For this review, use the dimensioned drawing (mm, ordinates from the lowest corner) and the shaded views. Coordinates: 2 decimals unless noted, no trailing zeros. Order: outer loops, then holes, each group sorted by start corner. A loop starts at its lowest first (then second) coordinate and runs counter-clockwise, first axis right, second up. Notation, with made-up numbers: (-33, -38.5) -> (10, -38.5) arc R31 cw to (10, -3.5) -> close; hole circle Ø9 at (64, -7). An arc over 180 degrees is marked (long way). Use one line per item in the form item = value. Start each with the question number.
(1) Take a section at A-A (z = 13.75). State the section outline as (x, y) points, then the cut area to 3 significant figures.
(2) Wall thickness on line 1 along X through (y, z) = (4, 24); line 2 along Z through (x, y) = (1.6, 4.6); line 3 along X through (y, z) = (1.9, 4.75): over which ranges is each line inside the solid? List them lowest first.
(3) Insertion check: pin 1 Ø3 at (y, z) = (2, 14.5) entering from -X; pin 2 Ø1 at (x, z) = (1.5, 21) entering from -Y. Each pin has a flat end and moves straight along its axis. Give the tip position at first contact, or say it passes through.
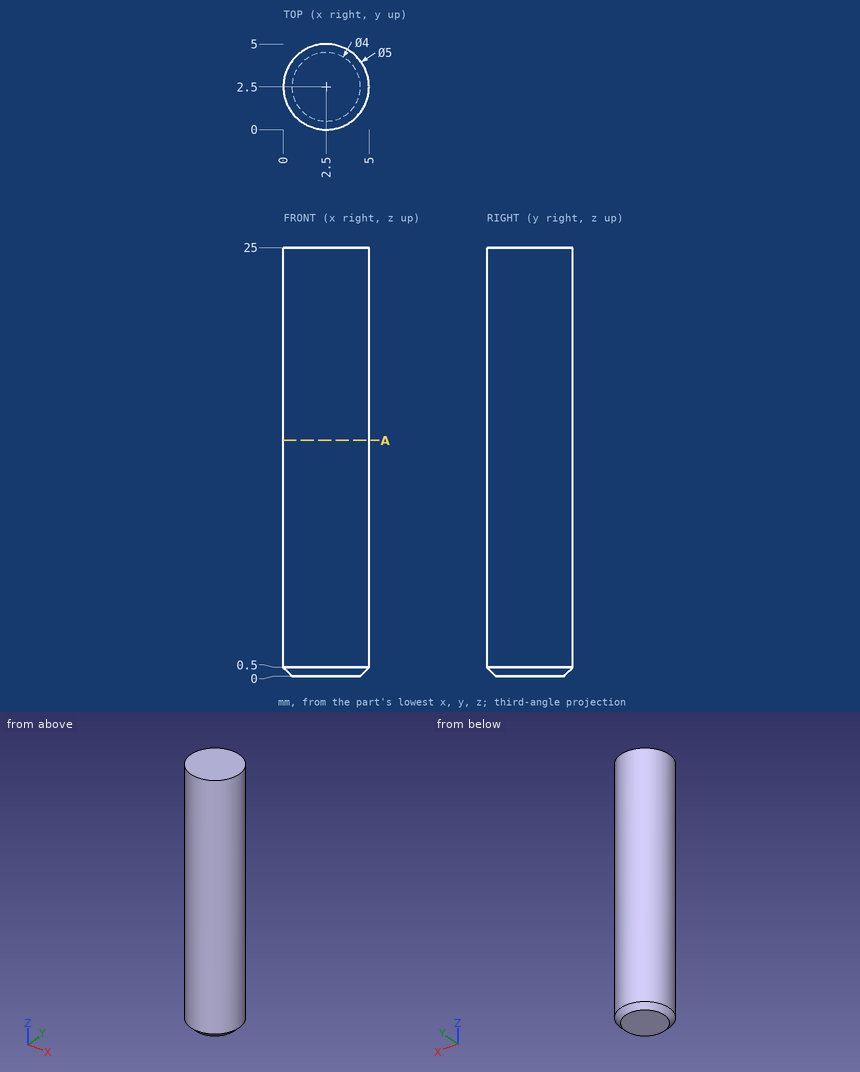
Findings:
q1.outline = circle Ø5 at (2.5, 2.5)
q1.area = 19.6 mm²
q2.line_1 = 0.5 to 4.5
q2.line_2 = 0.28 to 25
q2.line_3 = 0.07 to 4.93
q3.pin_1 = 0
q3.pin_2 = 0.05
